from build123d import *

# Parameters (mm, degrees)
CROQUIS1_R              = 1.35255
CROQUIS1_R_2            = 1.778
SALIENTE_EXTRUIR1_DEPTH = 3.175
CROQUIS5_R              = 2.55
CORTAR_EXTRUIR1_DEPTH   = 53.649355209
CROQUIS6_R              = 2.078
CROQUIS6_R_2            = 1.65255
CROQUIS6_R_3            = 2.85
CORTAR_EXTRUIR2_DEPTH   = 53.649355209


with BuildPart() as part:
    # Croquis1 → Saliente-Extruir1 (new body)
    with BuildSketch(Plane.XZ):
        with BuildLine():
            Line((-6.02234, -19.2405), (-6.02234, -20.828))
            ThreePointArc((-6.02234, -20.828), (-5.836352806, -21.277012806), (-5.38734, -21.463))
            Line((-5.38734, -21.463), (0.96266, -21.463))
            ThreePointArc((0.96266, -21.463), (1.411672806, -21.277012806), (1.59766, -20.828))
            Line((1.59766, -20.828), (1.59766, -19.2405))
            ThreePointArc((1.59766, -19.2405), (2.062627985, -18.117967985), (3.18516, -17.653))
            Line((3.18516, -17.653), (36.43122, -17.653))
            ThreePointArc((36.43122, -17.653), (41.454190356, -15.572417555), (43.534772801, -10.549447199))
            Line((43.534772801, -10.549447199), (43.534772801, 10.549447199))
            ThreePointArc((43.534772801, 10.549447199), (41.454190356, 15.572417555), (36.43122, 17.653))
            Line((36.43122, 17.653), (3.18516, 17.653))
            ThreePointArc((3.18516, 17.653), (2.062627985, 18.117967985), (1.59766, 19.2405))
            Line((1.59766, 19.2405), (1.59766, 20.828))
            ThreePointArc((1.59766, 20.828), (1.411672806, 21.277012806), (0.96266, 21.463))
            Line((0.96266, 21.463), (-5.38734, 21.463))
            ThreePointArc((-5.38734, 21.463), (-5.836352806, 21.277012806), (-6.02234, 20.828))
            Line((-6.02234, 20.828), (-6.02234, 19.2405))
            ThreePointArc((-6.02234, 19.2405), (-6.487307985, 18.117967985), (-7.60984, 17.653))
            Line((-7.60984, 17.653), (-23.755604, 17.653))
            ThreePointArc((-23.755604, 17.653), (-24.878136015, 18.117967985), (-25.343104, 19.2405))
            Line((-25.343104, 19.2405), (-25.343104, 20.828))
            ThreePointArc((-25.343104, 20.828), (-25.529091194, 21.277012806), (-25.978104, 21.463))
            Line((-25.978104, 21.463), (-32.328104, 21.463))
            ThreePointArc((-32.328104, 21.463), (-32.777116806, 21.277012806), (-32.963104, 20.828))
            Line((-32.963104, 20.828), (-32.963104, 19.2405))
            ThreePointArc((-32.963104, 19.2405), (-33.428071985, 18.117967985), (-34.550604, 17.653))
            Line((-34.550604, 17.653), (-36.43122, 17.653))
            ThreePointArc((-36.43122, 17.653), (-44.591052878, 14.273086555), (-47.970966323, 6.113253677))
            Line((-47.970966323, 6.113253677), (-47.970966323, -6.113253677))
            ThreePointArc((-47.970966323, -6.113253677), (-44.591052878, -14.273086555), (-36.43122, -17.653))
            Line((-36.43122, -17.653), (-34.550604, -17.653))
            ThreePointArc((-34.550604, -17.653), (-33.428071985, -18.117967985), (-32.963104, -19.2405))
            Line((-32.963104, -19.2405), (-32.963104, -20.828))
            ThreePointArc((-32.963104, -20.828), (-32.777116806, -21.277012806), (-32.328104, -21.463))
            Line((-32.328104, -21.463), (-25.978104, -21.463))
            ThreePointArc((-25.978104, -21.463), (-25.529091194, -21.277012806), (-25.343104, -20.828))
            Line((-25.343104, -20.828), (-25.343104, -19.2405))
            ThreePointArc((-25.343104, -19.2405), (-24.878136015, -18.117967985), (-23.755604, -17.653))
            Line((-23.755604, -17.653), (-7.60984, -17.653))
            ThreePointArc((-7.60984, -17.653), (-6.487307985, -18.117967985), (-6.02234, -19.2405))
        make_face()
        with Locations(Location((33.655, -7.874, 0), (0, 0, 90))):
            Circle(CROQUIS1_R, mode=Mode.SUBTRACT)
        with Locations(Location((-33.655, 7.874, 0), (0, 0, 90))):
            Circle(CROQUIS1_R, mode=Mode.SUBTRACT)
        with Locations(Location((-33.655, -7.874, 0), (0, 0, 90))):
            Circle(CROQUIS1_R, mode=Mode.SUBTRACT)
        with Locations(Location((-2.21234, 18.288, 0), (0, 0, 90))):
            Circle(CROQUIS1_R_2, mode=Mode.SUBTRACT)
        with Locations(Location((-29.153104, -18.288, 0), (0, 0, 90))):
            Circle(CROQUIS1_R_2, mode=Mode.SUBTRACT)
        with Locations(Location((-2.21234, -18.288, 0), (0, 0, 90))):
            Circle(CROQUIS1_R_2, mode=Mode.SUBTRACT)
        with Locations(Location((-29.153104, 18.288, 0), (0, 0, 90))):
            Circle(CROQUIS1_R_2, mode=Mode.SUBTRACT)
        with Locations(Location((33.655, 7.874, 0), (0, 0, 90))):
            Circle(CROQUIS1_R, mode=Mode.SUBTRACT)
        with BuildLine():
            Line((-33.9725, 2.4765), (-29.845, 2.4765))
            Line((-29.845, 2.4765), (-29.845, 9.645968035))
            ThreePointArc((-29.845, 9.645968035), (-31.52653105, 12.388525412), (-29.08046, 14.478))
            Line((-29.08046, 14.478), (29.08046, 14.478))
            ThreePointArc((29.08046, 14.478), (31.52653105, 12.388525412), (29.845, 9.645968035))
            Line((29.845, 9.645968035), (29.845, 2.4765))
            Line((29.845, 2.4765), (33.9725, 2.4765))
            ThreePointArc((33.9725, 2.4765), (36.449, 0), (33.9725, -2.4765))
            Line((33.9725, -2.4765), (29.845, -2.4765))
            Line((29.845, -2.4765), (29.845, -9.645968035))
            ThreePointArc((29.845, -9.645968035), (31.52653105, -12.388525412), (29.08046, -14.478))
            Line((29.08046, -14.478), (-29.08046, -14.478))
            ThreePointArc((-29.08046, -14.478), (-31.52653105, -12.388525412), (-29.845, -9.645968035))
            Line((-29.845, -9.645968035), (-29.845, -2.4765))
            Line((-29.845, -2.4765), (-33.9725, -2.4765))
            ThreePointArc((-33.9725, -2.4765), (-36.449, 0), (-33.9725, 2.4765))
        make_face(mode=Mode.SUBTRACT)
    extrude(amount=-SALIENTE_EXTRUIR1_DEPTH)

    # Croquis5 → Cortar-Extruir1 (cut, through all)
    with BuildSketch(Plane(origin=(0, 3.175, 0), x_dir=(1, 0, 0), z_dir=(0, 1, 0))):
        with Locations(Location((-42.138904379, 0, 0), (0, 0, 270))):
            Circle(CROQUIS5_R)
    extrude(amount=-CORTAR_EXTRUIR1_DEPTH, mode=Mode.SUBTRACT)

    # Croquis6 → Cortar-Extruir2 (cut, through all)
    with BuildSketch(Plane(origin=(0, 3.175, 0), x_dir=(1, 0, 0), z_dir=(0, 1, 0))):
        with Locations(Location((-29.153104, 18.288, 0), (0, 0, 270))):
            Circle(CROQUIS6_R)
        with Locations(Location((-33.655, 7.874, 0), (0, 0, 270))):
            Circle(CROQUIS6_R_2)
        with Locations(Location((-33.655, -7.874, 0), (0, 0, 270))):
            Circle(CROQUIS6_R_2)
        with Locations(Location((-29.153104, -18.288, 0), (0, 0, 270))):
            Circle(CROQUIS6_R)
        with Locations(Location((-2.21234, -18.288, 0), (0, 0, 270))):
            Circle(CROQUIS6_R)
        with Locations(Location((-42.138904379, 0, 0), (0, 0, 270))):
            Circle(CROQUIS6_R_3)
        with Locations(Location((-2.21234, 18.288, 0), (0, 0, 270))):
            Circle(CROQUIS6_R)
        with Locations(Location((33.655, 7.874, 0), (0, 0, 270))):
            Circle(CROQUIS6_R_2)
        with Locations(Location((33.655, -7.874, 0), (0, 0, 270))):
            Circle(CROQUIS6_R_2)
    extrude(amount=-CORTAR_EXTRUIR2_DEPTH, mode=Mode.SUBTRACT)


solid = part.part
Model file for the job. Use its own axes, mm. A direction names the side the tool comes from. Give positions to 0.01 mm unless a question says otherwise; leave off trailing zeros. Loops run counter-clockwise (first coordinate to the right, second up) from the corner with the lowest first, then second, coordinate; pieces in that order, holes last. Notation, with made-up numbers: (61, 37) -> (102, 37) arc R26 ccw to (102, 72) -> close; hole circle Ø7 at (46, 14). An arc over 180 degrees is marked (long way). Use a Markdown table: item, result. Add a question column.
(1) Slice it at B-B on x = 25. List the corners of the cut face in (y, z) (3 decimals).
(2) Drop flat-ended pins along their axis: pin 1 Ø1.7 at (y, z) = (1.5, -20.5) entering from -X; pin 2 Ø4.5 at (x, z) = (-33.655, -7.874) entering from +Y (3 decimals); pin 3 Ø3 at (x, z) = (33.655, 7.874) entering from -Y; pin 4 Ø1.3 at (y, z) = (1.5, 20) entering from +X. Give the stop position or say it passes through.
(3) Slice it at A-A on z = 0. List the corners of the cut face in (x, y) (3 decimals), and give its area (3 significant figures).
(4) Wall check: line 1 along Z through (x, y) = (1, 0.2); line 2 along Z through (x, y) = (19, 1.05); line 3 along X through (y, z) = (2.2, 7.5) (3 decimals). Give the ranges that are in metal, low to high.
(5) Mould opens along Z. For faces 1 (the flat face through (-2, 2, 21.463)), 2 (the cylindrical face through (35.3, 1.6, 7.7)), 3 (the flat face through (-6.022, 2, 20)) say: +Z half, -Z half, draft (parallel to the pull), parting line (faces both ways), or undercut.
(6) Slice it at C-C on y = 2.4. Give the number of separate pieces and of enclosed holes in the cut face, and give its area (3 significant figures).
(7) Tool access for faces 4 (the cylindrical face through (31.534, 1.565, -12.34)), 5 (the flat face through (-25.343, 2, 20)), 6 (the flat face through (-25.343, 2, -20)), 7 (the flat face through (20, 2, 17.653)), 8 (the cylindrical face through (41.399, 1.565, -15.627)): list every direction of +Z, -Z, +X, -X, +Y, -Y with a clear straight run to the whole face (end or side of a thin tool).
Filled sheet:
| question | item | result |
|---|---|---|
| 1 | outline | (0, -17.653) -> (3.175, -17.653) -> (3.175, -14.478) -> (0, -14.478) -> close; (0, 14.478) -> (3.175, 14.478) -> (3.175, 17.653) -> (0, 17.653) -> close |
| 2 | pin 1 | x = -32.96 |
| 2 | pin 2 | y = 3.175 |
| 2 | pin 3 | through |
| 2 | pin 4 | x = 1.6 |
| 3 | outline | (-47.971, 0) -> (-44.989, 0) -> (-44.989, 3.175) -> (-47.971, 3.175) -> close; (-39.289, 0) -> (-36.449, 0) -> (-36.449, 3.175) -> (-39.289, 3.175) -> close; (36.449, 0) -> (43.535, 0) -> (43.535, 3.175) -> (36.449, 3.175) -> close |
| 3 | area | 41.0 mm2 |
| 4 | line 1 | -21.46 to -14.48, 14.48 to 21.46 |
| 4 | line 2 | -17.65 to -14.48, 14.48 to 17.65 |
| 4 | line 3 | -47.887 to -35.265, -32.045 to -29.845, 29.845 to 32.045, 35.265 to 43.535 |
| 5 | face 1 | +Z half |
| 5 | face 2 | undercut |
| 5 | face 3 | draft |
| 6 | separate pieces | 1 |
| 6 | enclosed holes | 10 |
| 6 | area | 1,350 mm2 |
| 7 | face 4 | +Y, -Y |
| 7 | face 5 | +Z, +Y, -Y |
| 7 | face 6 | -Z, +Y, -Y |
| 7 | face 7 | +Z, +X, +Y, -Y |
| 7 | face 8 | -Z, +X, +Y, -Y |
